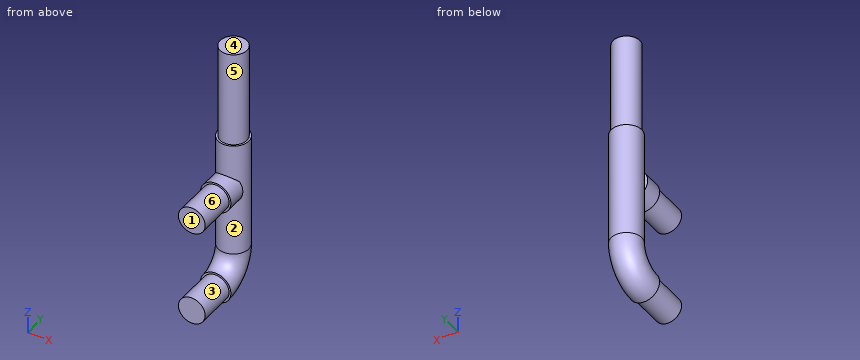
Autodesk Inventor part; units mm, degrees
ref_plane "Work Plane1" through (0, -7.5, 0) normal (0, 1, 0) x (-1, 0, 0)
ref_plane "Work Plane2" through (0, 0, 17.5) normal (0, 0, 1) x (1, 0, 0)
ref_plane "YZ Plane" through (0, 0, 0) normal (1, 0, 0) x (0, 1, 0)
sketch "Sketch2" plane through (0, 0, 0) normal (0, 0, 1) x (1, 0, 0)
  circle A0 centre (0, 0) radius 4
  dimension "d0" = 8
ref_plane "Work Plane1" through (0, -7.5, 0) normal (0, 1, 0) x (-1, 0, 0)
sketch "Sketch3" plane through (0, -7.5, 0) normal (0, 1, 0) x (-1, 0, 0)
  circle A0 centre (0, -7.5) radius 4
  line L0 (5.6, 0) -> (-5.6, 0)
  point P0 (0, 0)
  dimension "d2" = 8
  dimension "d3" = 7.5
revolve "Revolution1" add sketch "Sketch3" angle 90 about axis through (-10, -7.5, 0) along (1, 0, 0)
extrude "Extrusion1" add sketch "Sketch2" along normal blind 17.5
sketch "Sketch4" plane through (0, 0, 17.5) normal (0, 0, 1) x (1, 0, 0)
  circle A0 centre (0, 0) radius 4
  dimension "d7" = 8
ref_plane "Work Plane2" through (0, 0, 17.5) normal (0, 0, 1) x (1, 0, 0)
extrude "Extrusion2" add sketch "Sketch4" along normal blind 12.5
sketch "Sketch5" plane through (0, -7.5, 0) normal (0, 1, 0) x (-1, 0, 0)
  circle A0 centre (0, 17.5) radius 4
  line L0 (-10.5, 17.5) -> (10.5, 17.5)
  point P0 (0, 0)
  dimension "d11" = 8
  dimension "d12" = 0
extrude "Extrusion3" add sketch "Sketch5" along normal blind 5
sketch "Sketch7" plane through (0, -7.5, -7.5) normal (0, -1, 0) x (1, 0, 0)
  circle A0 centre (0, 0) radius 3.5
  point P0 (0, 7.5)
  dimension "d18" = 7
extrude "Extrusion4" add sketch "Sketch7" along normal blind 10
sketch "Sketch8" plane through (0, -7.5, 0) normal (0, -1, 0) x (1, 0, 0)
  circle A0 centre (0, 17.5) radius 3.5
  circle A1 centre (0, -7.5) radius 3.5
  point P0 (0, 0)
  dimension "d21" = 7
  dimension "d22" = 25
extrude "Extrusion5" add sketch "Sketch8" along normal blind 10 contours A0
sketch "Sketch10" plane through (0, 0, 30) normal (0, 0, 1) x (1, 0, 0)
  circle A0 centre (0, 0) radius 4
  circle A1 centre (0, 0) radius 3.5
  dimension "d29" = 7
extrude "Extrusion7" add sketch "Sketch10" along normal mid plane 50 contours A1
properties part number "1p10 DP3 roller attachment final"
Verification items for the finished model (mm, model axes). Face numbers are marked on the shaded views. A direction names the side the tool comes from. Coordinates: 2 decimals unless noted, no trailing zeros. Order: outer loops, then holes, each group sorted by start corner. A loop starts at its lowest first (then second) coordinate and runs counter-clockwise, first axis right, second up.
1. Go/stop test with flat-tipped pins: pin 1 Ø0.7 at (x, z) = (-3.5, 18) entering from +Y; pin 2 Ø2 at (x, y) = (-2.5, -10.5) entering from +Z; pin 3 Ø3 at (x, z) = (-2, 43) entering from -Y. Record where each tip stops, or that it passes through.
Results found:
pin 1: stops at y = 2.47
pin 2: stops at z = 20.66
pin 3: stops at y = -3.46
2. Sectioned sample at D-D, the plane z = 26.5. Record the cut outline in (x, y), and give its area (3 significant figures).
Results found:
outline: circle Ø8 at (0, 0)
area: 50.3 mm2
3. Sectioned sample at C-C, the plane x = 0. Record the cut outline in (y, z), and give its area (3 significant figures).
Results found:
outline: (-17.5, -11) - (-7.5, -11) - (-7.5, -11.5) arc R11.5 ccw to (4, 0) - (4, 30) - (3.5, 30) - (3.5, 55) - (-3.5, 55) - (-3.5, 30) - (-4, 30) - (-4, 21.5) - (-7.5, 21.5) - (-7.5, 21) - (-17.5, 21) - (-17.5, 14) - (-7.5, 14) - (-7.5, 13.5) - (-4, 13.5) - (-4, 0) arc R3.5 cw to (-7.5, -3.5) - (-7.5, -4) - (-17.5, -4) - close
area: 677 mm2
4. Scan lines: line 1 (Z direction, x = -1.25, y = -10.75); line 2 (Y direction, x = -0.25, z = 28.5); line 3 (Z direction, x = 2.5, y = -11.5). Record each from-to range of solid material in increasing order.
Results found:
line 1: z = -10.77 to -4.23, 14.23 to 20.77
line 2: y = -3.99 to 3.99
line 3: z = -9.95 to -5.05, 15.05 to 19.95
5. Sectioned sample at B-B, the plane y = -13.5. Record the cut outline in (x, z).
Results found:
outline: circle Ø7 at (0, -7.5); circle Ø7 at (0, 17.5)
6. Release check for a two-part mould opening along Z. For the marked faces 4, 5 and 6 record: +Z half, -Z half, draft (parallel to the pull), parting line (faces both ways), or undercut.
Results found:
face 4: +Z half
face 5: draft
face 6: undercut
7. Set-up check for the marked faces 1, 2 and 3: record each of +Z, -Z, +X, -X, +Y, -Y from which the full face is reachable in a straight line by a thin tool's end or side.
Results found:
face 1: +Z, -Z, +X, -X, -Y
face 2: none
face 3: -Y
8. Sectioned sample at A-A, the plane z = 17.5. Record the cut outline in (x, y), and give its area (3 significant figures).
Results found:
outline: (-4, -7.5) - (-3.5, -7.5) - (-3.5, -17.5) - (3.5, -17.5) - (3.5, -7.5) - (4, -7.5) - (4, -2.5) - (3.12, -2.5) arc R4 ccw (long way) to (-3.12, -2.5) - (-4, -2.5) - close
area: 154 mm2
